Here's how the part is built. I have some questions about the finished solid (model axes, mm). Face numbers are marked on the shaded views. A direction names the side the tool comes from. Round coordinates to 2 decimals unless told otherwise and drop trailing zeros. Order: outer loops, then holes, each group sorted by start corner. A loop starts at its lowest first (then second) coordinate and runs counter-clockwise, first axis right, second up. Notation, with made-up numbers: M 10,-18.5 L 55,-18.5 A21 cw 55,14.5 Z; hole C 75,81.5 d7. An arc over 180 degrees is marked long. Write item = value, one per line. Start each with the question number.
Item 1: I want a section at D-D, the plane x = 14. List the corners of the cut face in (y, z) for me.
Item 2: Please list where these lines run through material, in increasing order: L1, parallel to Z at x = 0, y = 2 (3 decimals); L2, parallel to Y at x = 8, z = -2.5.
Item 3: I want a section at B-B, the plane z = 0. List the corners of the cut face in (x, y) for me (3 decimals).
Item 4: I want a section at A-A, the plane x = 0. List the corners of the cut face in (y, z) for me (3 decimals), plus the area to 3 significant figures.
Item 5: For the marked faces 1 and 2, which set-ups out of +Z, -Z, +X, -X, +Y, -Y let a thin tool reach every point of the face, with its end or its side?
Item 6: I want a section at C-C, the plane y = 58.5. List the corners of the cut face in (x, z) for me (3 decimals), plus the area to 3 significant figures.
Item 7: I'm going to push flat-ended pins straight in: P1, Ø8, axis at y = 60, z = -13, coming from the +X side (3 decimals); P2, Ø5, axis at x = 0.5, y = 57.5, coming from the -Z side; P3, Ø12, axis at x = -9.5, z = -7, coming from the +Y side. Where does each tip first touch, or does it pass through?
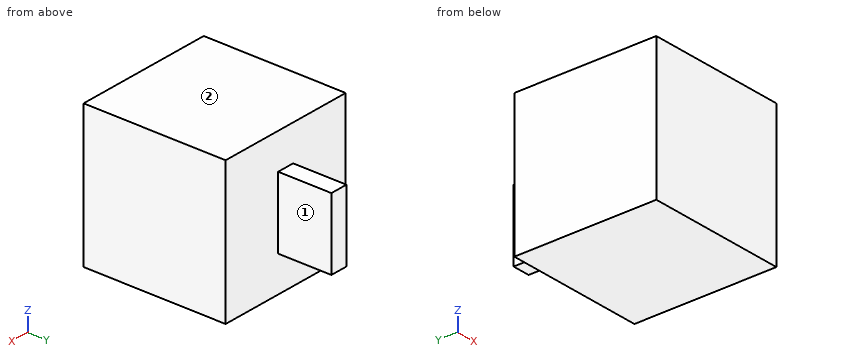
Autodesk Inventor part; units mm, degrees
ref_plane "YZ Plane" through (0, 0, 0) normal (1, 0, 0) x (0, 1, 0)
ref_plane "XZ Plane" through (0, 0, 0) normal (0, 1, 0) x (-1, 0, 0)
ref_plane "XY Plane" through (0, 0, 0) normal (0, 0, 1) x (1, 0, 0)
sketch "Sketch1" plane through (0, 0, 0) normal (0, 1, 0) x (-1, 0, 0)
  line L0 (-25.4, -25.4) -> (25.4, -25.4)
  line L1 (25.4, -25.4) -> (25.4, 25.4)
  line L2 (25.4, 25.4) -> (-25.4, 25.4)
  line L3 (-25.4, 25.4) -> (-25.4, -25.4)
  point P0 (0, 0)
  dimension "d0" = 50.8
  dimension "d1" = 50.8
extrude "Extrusion1" add sketch "Sketch1" along normal blind 2.794
sketch "Sketch2" plane through (0, 2.794, 0) normal (0, 1, 0) x (1, 0, 0)
  circle A0 centre (0, 0) radius 10.795
  dimension "d4" = 21.59
extrude "Extrusion2" cut sketch "Sketch2" against normal blind 2.54
sketch "Sketch3" plane through (0, 2.794, 0) normal (0, 1, 0) x (1, 0, 0)
  point P0 (0, 0)
sketch "Sketch4" plane through (0, 2.794, 0) normal (0, 1, 0) x (1, 0, 0)
  line L0 (25.4, 25.4) -> (-25.4, 25.4)
  line L1 (-25.4, -25.4) -> (25.4, -25.4)
  line L2 (25.4, 25.4) -> (-25.4, 25.4)
  line L3 (-25.4, 25.4) -> (-25.4, -25.4)
  line L4 (-25.4, -25.4) -> (25.4, -25.4)
  line L5 (25.4, -25.4) -> (25.4, 25.4)
  point P0 (0, 0)
extrude "Extrusion3" add sketch "Sketch4" along normal blind 48.006
sketch "Sketch5" plane through (0, 50.8, 0) normal (0, 1, 0) x (1, 0, 0)
  line L0 (3.175, 12.7) -> (-3.175, 12.7)
  line L1 (-3.175, 12.7) -> (-3.175, -12.7)
  line L2 (-3.175, -12.7) -> (3.175, -12.7)
  line L3 (3.175, -12.7) -> (3.175, 12.7)
  point P0 (0, 0)
  dimension "d9" = 6.35
  dimension "d10" = 25.4
extrude "Extrusion4" add sketch "Sketch5" along normal blind 19.05
properties part number "block for magnet"
Filled in:
q1.outline = M 0,-25.4 L 50.8,-25.4 L 50.8,25.4 L 0,25.4 Z
q2.L1 = -25.4 to -10.795, 10.795 to 25.4
q2.L2 = 0 to 0.25, 2.79 to 50.8
q3.outline = M -25.4,0 L 25.4,0 L 25.4,50.8 L 3.175,50.8 L 3.175,69.85 L -3.175,69.85 L -3.175,50.8 L -25.4,50.8 Z; hole M -10.795,0.254 L 10.795,0.254 L 10.795,2.794 L -10.795,2.794 Z
q4.outline = M 0,-25.4 L 50.8,-25.4 L 50.8,-12.7 L 69.85,-12.7 L 69.85,12.7 L 50.8,12.7 L 50.8,25.4 L 0,25.4 Z; hole M 0.254,-10.795 L 2.794,-10.795 L 2.794,10.795 L 0.254,10.795 Z
q4.area = 3,010 mm^2
q5.face_1 = +Z, -Z, +X, +Y
q5.face_2 = +Z, +X, -X, +Y, -Y
q6.outline = M -3.175,-12.7 L 3.175,-12.7 L 3.175,12.7 L -3.175,12.7 Z
q6.area = 161 mm^2
q7.P1 = 3.175
q7.P2 = -12.7
q7.P3 = 50.8
